```python
from build123d import *

# Parameters (mm, degrees)
BOSS_EXTRUDE1_DEPTH = 31.5
SKETCH5_R           = 5
CUT_EXTRUDE1_DEPTH  = 25


with BuildPart() as part:
    # Sketch1 → Boss-Extrude1 (new body)
    with BuildSketch(Plane(origin=(0, 0, 0), x_dir=(1, 0, 0), z_dir=(0, 1, 0))):
        with BuildLine():
            ThreePointArc((-1.048467756, 7.218012428), (-2.699998527, 12.414164851), (-7.048467756, 15.703293803))
            ThreePointArc((-7.048467756, 15.703293803), (-10.048467756, 16.218012428), (-13.048467756, 15.703293803))
            ThreePointArc((-13.048467756, 15.703293803), (-15.244620178, -0.1304568), (-1.048467756, 7.218012428))
        make_face()
        with BuildLine():
            ThreePointArc((-13.048467756, 15.703293803), (-10.048467756, 16.218012428), (-7.048467756, 15.703293803))
            Line((-7.048467756, 15.703293803), (-7.048467756, 19.203293803))
            Line((-7.048467756, 19.203293803), (-13.048467756, 19.203293803))
            Line((-13.048467756, 19.203293803), (-13.048467756, 15.703293803))
        make_face()
    extrude(amount=BOSS_EXTRUDE1_DEPTH)

    # Sketch5 → Cut-Extrude1 (cut)
    with BuildSketch(Plane(origin=(0, 31.5, 0), x_dir=(1, 0, 0), z_dir=(0, 1, 0))):
        with Locations((-10.048467756, 7.270239538)):
            Circle(SKETCH5_R)
    extrude(amount=-CUT_EXTRUDE1_DEPTH, mode=Mode.SUBTRACT)


solid = part.part
```
Check sheet for the modelled part. Datum: model origin and axes. Units: mm. A direction names the side the tool comes from. Coordinates: 2 decimals unless noted, no trailing zeros. Order: outer loops, then holes, each group sorted by start corner. A loop starts at its lowest first (then second) coordinate and runs counter-clockwise, first axis right, second up. Notation, with made-up numbers: (4, 89.25) -> (33, 89.25) arc R31 ccw to (33, 127.25) -> close; hole circle Ø4 at (-4, 54). An arc over 180 degrees is marked (long way). Write item = value, one per line. Start each with the question number.
1) Cross-section at A-A (z = -3.25). Enter the section's corners in (x, y), then the cut area to 3 significant figures.
2) Cross-section at C-C (y = 29.5). Enter the section's corners in (x, z).
3) Go/stop test with flat-tipped pins: P1, Ø1, axis at x = -16.5, y = 25.5, coming from the +Z side; P2, Ø1.5, axis at x = -13.5, y = 9.5, coming from the +Z side; P3, Ø5, axis at x = -3.5, y = 22.5, coming from the +Z side. Record where each tip stops, or that it passes through.
4) Access from +Z, -Z, +X, -X, +Y, -Y to the whole of each face (thin tool, end or side, straight path). Record for faces 1 (the flat face through (-7.048, 16, -17)), 2 (the flat face through (-10, 16, -19.203)), 3 (the cylindrical face through (-11.13, 19.18, -2.39)).
5) Mould release check, pull along X, two halves, no side actions. Record for faces 4 (the flat face through (-10, 0, -9)), 5 (the flat face through (-10, 6.5, -7)), 6 (the flat face through (-13.048, 16, -17)): +X half, -X half, draft (parallel to the pull), parting line (faces both ways), or undercut.
6) Cross-section at D-D (x = -3.75). Enter the section's corners in (y, z), then the cut area to 3 significant figures.
7) Cross-section at B-B (x = -11.5). Enter the section's corners in (y, z).
8) Material ranges on L1, parallel to Z at x = -10.25, y = 14.5; L2, parallel to X at y = 12, z = -7.5; L3, parallel to X at y = 28.5, z = -9.75, recorded low to high.
Ans:
q1.outline = (-18.13, 0) -> (-1.97, 0) -> (-1.97, 31.5) -> (-7.08, 31.5) -> (-7.08, 6.5) -> (-13.02, 6.5) -> (-13.02, 31.5) -> (-18.13, 31.5) -> close
q1.area = 360 mm²
q2.outline = (-13.05, -19.2) -> (-7.05, -19.2) -> (-7.05, -15.7) arc R9 ccw (long way) to (-13.05, -15.7) -> close; hole circle Ø10 at (-10.05, -7.27)
q3.P1 = -0.47
q3.P2 = 1.37
q3.P3 = 0.82
q4.face_1 = -Z, +X, +Y, -Y
q4.face_2 = -Z, +X, -X, +Y, -Y
q4.face_3 = +Y
q5.face_4 = draft
q5.face_5 = undercut
q5.face_6 = -X half
q6.outline = (0, -13.65) -> (31.5, -13.65) -> (31.5, -0.79) -> (0, -0.79) -> close
q6.area = 405 mm²
q7.outline = (0, -19.2) -> (31.5, -19.2) -> (31.5, -12.05) -> (6.5, -12.05) -> (6.5, -2.49) -> (31.5, -2.49) -> (31.5, 1.66) -> (0, 1.66) -> close
q8.L1 = -19.2 to -12.27, -2.27 to 1.78
q8.L2 = -19.04 to -15.04, -5.05 to -1.05
q8.L3 = -18.68 to -14.39, -5.71 to -1.41
